```python
from build123d import *

# Parameters (mm, degrees)
SKETCH1_R                                        = 11.1125
EXTRUDE1_DEPTH                                   = 6.35
D_GAGEMENT_51_D                                  = 3.4544
TROU_POUR_TARAUDAGE_POUR_TROU_TARAUD_5_D         = 2.5781
CHAMBRAGE_POUR_VIS_T_TE_RONDE_BOMB_E_D           = 2.794
CHAMBRAGE_POUR_VIS_T_TE_RONDE_BOMB_E_CBORE_D     = 5.55752
CHAMBRAGE_POUR_VIS_T_TE_RONDE_BOMB_E_CBORE_DEPTH = 1.8034


with BuildPart() as part:
    # Sketch1 → Extrude1 (new body)
    with BuildSketch(Plane(origin=(0, 0, 0), x_dir=(1, 0, 0), z_dir=(0, 1, 0))):
        Circle(SKETCH1_R)
    extrude(amount=-EXTRUDE1_DEPTH)

    # Dégagement #51 (through all)
    with Locations(Plane(origin=(0, 0, 0), x_dir=(-1, 0, 0), z_dir=(0, 1, 0))):
        with Locations((7.9375, 0), (0, -7.9375), (-7.9375, 0), (0, 7.9375)):
            Hole(D_GAGEMENT_51_D / 2)

    # Trou pour taraudage pour trou taraudé #5-401 (through all)
    with Locations(Plane.XZ.offset(6.35)):
        with Locations((-5.612660076, -5.612660076), (5.612660076, -5.612660076), (5.612660076, 5.612660076), (-5.612660076, 5.612660076)):
            Hole(TROU_POUR_TARAUDAGE_POUR_TROU_TARAUD_5_D / 2)

    # Chambrage pour vis à tête ronde bombée #31 (through all)
    with Locations(Plane(origin=(0, 0, 0), x_dir=(-1, 0, 0), z_dir=(0, 1, 0))):
        with Locations((0, 0)):
            CounterBoreHole(CHAMBRAGE_POUR_VIS_T_TE_RONDE_BOMB_E_D / 2, CHAMBRAGE_POUR_VIS_T_TE_RONDE_BOMB_E_CBORE_D / 2, CHAMBRAGE_POUR_VIS_T_TE_RONDE_BOMB_E_CBORE_DEPTH)


solid = part.part
```
Source: CAD feature listing. Evaluate the final solid. Frame: model axes, mm. A direction names the side the tool comes from. Give positions to 0.01 mm unless a question says otherwise; leave off trailing zeros. Loops run counter-clockwise (first coordinate to the right, second up) from the corner with the lowest first, then second, coordinate; pieces in that order, holes last. Notation, with made-up numbers: (7, 57.25) - (63, 57.25) arc R26 cw to (63, 90.25) - close; hole circle Ø1 at (-15.75, 67). An arc over 180 degrees is marked (long way). Use CSV: the item, a comma, the result in double quotes.
1) Line query: line 1 (Z direction, x = 0, y = -4.5); line 2 (X direction, y = -4.5, z = 6.5); line 3 (X direction, y = -3.75, z = 0.5). Output: solid intervals per line, ascending.
Worked out:
line 1,"z = -11.11 to -9.66, -6.21 to -1.4, 1.4 to 6.21, 9.66 to 11.11"
line 2,"x = -9.01 to -6.55, -4.68 to -0.96, 0.96 to 4.68, 6.55 to 9.01"
line 3,"x = -11.1 to -9.59, -6.28 to -1.3, 1.3 to 6.28, 9.59 to 11.1"
2) Mould query, pull axis X, two halves, no side actions, for faces 1 (the cylindrical face through (6.212, -3.219, 0.076)), 2 (the cylindrical face through (10.6, -3.13, -3.34)), 3 (the flat face through (2.3, 0, 2.3)). Classes: +X half, -X half, draft (parallel to the pull), parting line (faces both ways), or undercut.
Worked out:
face 1,"undercut"
face 2,"parting line"
face 3,"draft"
3) Cut plane D-D (z = 9). Output: boundary loops of the cut face in (x, y), and give its area (3 significant figures).
Worked out:
outline,"(-6.52, -6.35) - (-1.36, -6.35) - (-1.36, 0) - (-6.52, 0) - close; (1.36, -6.35) - (6.52, -6.35) - (6.52, 0) - (1.36, 0) - close"
area,"65.5 mm^2"
4) Pin query (flat end, axial travel): P1, Ø4, axis at x = 0, z = 7.94, coming from the -Y side; P2, Ø2, axis at x = -6, y = -3, coming from the +Z side. Return the tip coordinate at first contact, or that it passes through.
Worked out:
P1,"stops at y = -6.35"
P2,"stops at z = 9.92"
5) Cut plane C-C (y = -1.5). Count the separate pieces of the cut face and the enclosed holes in it, and give its area (3 significant figures).
Worked out:
separate pieces,"1"
enclosed holes,"9"
area,"305 mm^2"
6) Set-up query: faces 4 (the cylindrical face through (-0.22, -3.22, 9.65)), 5 (the flat face through (-1.2, -1.803, -1.2)). Return all of +Z, -Z, +X, -X, +Y, -Y with unobstructed straight access to the full face (end or side cutting, diameter ignored); none if empty.
Worked out:
face 4,"+Y, -Y"
face 5,"+Y"
7) Cut plane A-A (z = 0). Output: boundary loops of the cut face in (x, y).
Worked out:
outline,"(-11.11, -6.35) - (-9.66, -6.35) - (-9.66, 0) - (-11.11, 0) - close; (-6.21, -6.35) - (-1.4, -6.35) - (-1.4, -1.8) - (-2.78, -1.8) - (-2.78, 0) - (-6.21, 0) - close; (1.4, -6.35) - (6.21, -6.35) - (6.21, 0) - (2.78, 0) - (2.78, -1.8) - (1.4, -1.8) - close; (9.66, -6.35) - (11.11, -6.35) - (11.11, 0) - (9.66, 0) - close"
8) Cut plane B-B (x = 0). Output: boundary loops of the cut face in (y, z).
Worked out:
outline,"(-6.35, -11.11) - (0, -11.11) - (0, -9.66) - (-6.35, -9.66) - close; (-6.35, -6.21) - (0, -6.21) - (0, -2.78) - (-1.8, -2.78) - (-1.8, -1.4) - (-6.35, -1.4) - close; (-6.35, 1.4) - (-1.8, 1.4) - (-1.8, 2.78) - (0, 2.78) - (0, 6.21) - (-6.35, 6.21) - close; (-6.35, 9.66) - (0, 9.66) - (0, 11.11) - (-6.35, 11.11) - close"
